Geometry check sheet. Reference: drawing and pictorial views, mm from the part's lowest x, y, z. Give positions to 0.01 mm unless a question says otherwise; leave off trailing zeros. Loops run counter-clockwise (first coordinate to the right, second up) from the corner with the lowest first, then second, coordinate; pieces in that order, holes last. Notation, with made-up numbers: (17.25, -23.75) - (71.25, -23.75) arc R26 ccw to (71.25, -4.75) - close; hole circle Ø5 at (-4, 28). An arc over 180 degrees is marked (long way). One line per question, with ' | ' between items. Start each with the question number.
1. Section check A-A, the plane y = 3. Enter the section's corners in (x, z), then the cut area to 3 significant figures.
2. Section check C-C, the plane x = 5.5. Enter the section's corners in (y, z).
3. Section check D-D, the plane y = 7. Enter the section's corners in (x, z).
4. Section check B-B, the plane z = 0.55. Enter the section's corners in (x, y).
5. Depth check by flat-ended pin: pin 1 Ø0.8 at (x, z) = (5, 1.5) entering from -Y; pin 2 Ø0.9 at (y, z) = (8, 1) entering from +X; pin 3 Ø0.5 at (x, z) = (0.5, 1.5) entering from +Y. Enter the tip coordinate at first touch or a pass-through.
6. Thickness scan on line 1 along Z through (x, y) = (4, 8); line 2 along Y through (x, z) = (11.25, 0.65); line 3 along Y through (x, z) = (5.25, 1.55). Record the ranges inside material, lowest first. Write a range as from..to.
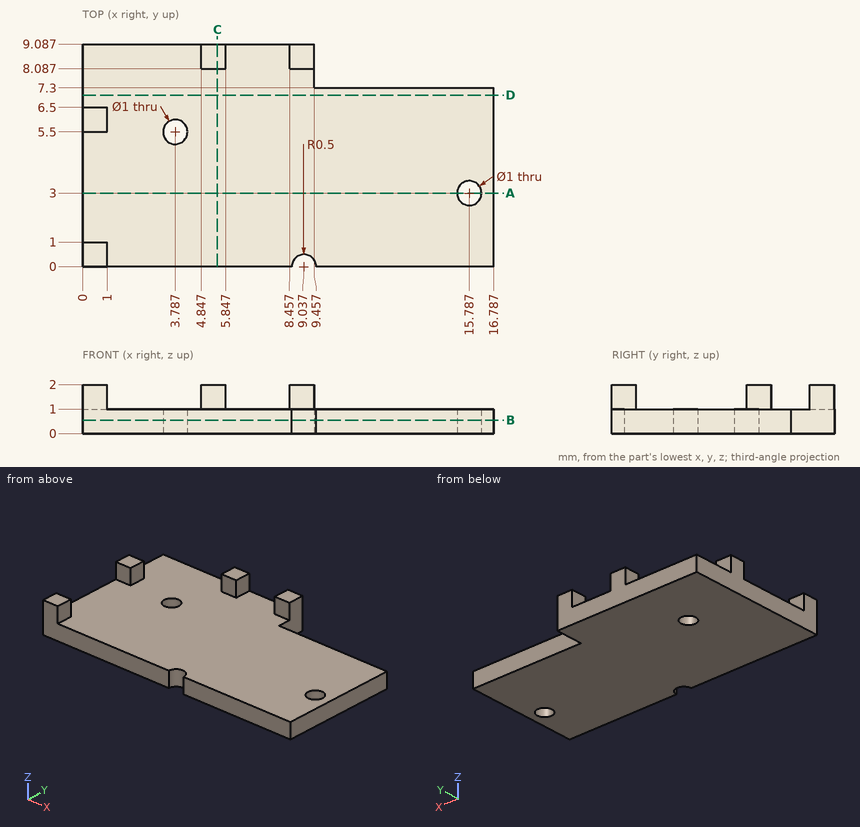
Results list:
1) outline: (0, 0) - (15.29, 0) - (15.29, 1) - (0, 1) - close; (16.29, 0) - (16.79, 0) - (16.79, 1) - (16.29, 1) - close | area: 15.8 mm²
2) outline: (0, 0) - (9.09, 0) - (9.09, 2) - (8.09, 2) - (8.09, 1) - (0, 1) - close
3) outline: (0, 0) - (16.79, 0) - (16.79, 1) - (0, 1) - close
4) outline: (0, 0) - (8.54, 0) arc R0.5 cw to (9.54, 0) - (16.79, 0) - (16.79, 7.3) - (9.46, 7.3) - (9.46, 9.09) - (0, 9.09) - close; hole circle Ø1 at (3.79, 5.5); hole circle Ø1 at (15.79, 3)
5) pin 1: y = 8.09 | pin 2: x = 9.46 | pin 3: y = 6.5
6) line 1: 0..1 | line 2: 0..7.3 | line 3: 8.09..9.09
